Input: part model. Units: mm. Frame: model coordinates. Round coordinates to 2 decimals unless told otherwise and drop trailing zeros. Order: outer loops, then holes, each group sorted by start corner. A loop starts at its lowest first (then second) coordinate and runs counter-clockwise, first axis right, second up. Notation, with made-up numbers: (-35, 53) -> (-11, 53) arc R16 cw to (-11, 58) -> close; hole circle Ø3 at (25.5, 34). An arc over 180 degrees is marked (long way). Answer as CSV lines item,"result". Start each with the question number.
1) Section query C-C, the plane y = 15. Output: boundary loops of the cut face in (x, z).
2) Mould query, pull axis Z, two halves, no side actions, for faces 1 (the face through (-2.71, 50.7, 12.203)), 2 (the face through (10, 50.6, -3.2)). Classes: +Z half, -Z half, draft (parallel to the pull), parting line (faces both ways), or undercut.
3) Section query B-B, the plane x = 0. Output: boundary loops of the cut face in (y, z), and give its area (3 significant figures).
4) Section query A-A, the plane z = 0. Output: boundary loops of the cut face in (x, y).
5) Line query: L1, parallel to X at y = 40, z = 0; L2, parallel to Z at x = 6.5, y = 59.5. Output: solid intervals per line, ascending.
6) First-contact query: P1, Ø2, axis at x = -8, z = 3.5, coming from the +Y side; P2, Ø5, axis at x = -5.5, y = 51.5, coming from the +Z side; P3, Ø2, axis at x = -6.5, y = 54.5, coming from the +Z side (3 decimals); P4, Ø6, axis at y = 13.5, z = 0.5, coming from the +X side. Flat tips, straight axial feed; report the tip coordinate or a pass-through.
Solid Edge part; units mm, degrees
sketch "Sketch1" plane through (0, 0, 0) normal (0, 0, 1) x (1, 0, 0)
  line L0 (0, 0) -> (0, 100)
sketch "Sketch2" plane through (0, 0, 0) normal (0, -1, 0) x (1, 0, 0)
  circle A0 centre (0, 0) radius 12.5
sweep "SweptProtrusion_1" add profiles "Sketch2" path "Sketch1"
shell "Thinwall_1" thickness 2 removed faces 2 at (-8.0833, 0, 8.5833) at (-8.0833, 100, 8.5833)
sketch "Sketch3" plane through (0, 0, 0) normal (1, 0, 0) x (0, 1, 0)
  circle A0 centre (0, 0) radius 12.5
  circle A1 centre (100, 0) radius 12.5
extrude "Cutout1" cut sketch "Sketch3" along normal through all and the other way through all
properties material "Stainless steel"
Findings:
1,outline,"circle Ø25 at (0, 0); hole circle Ø21 at (0, 0)"
2,face 1,"parting line"
2,face 2,"undercut"
3,outline,"(0, -12.5) -> (100, -12.5) arc R12.5 cw to (93.22, -10.5) -> (6.78, -10.5) arc R12.5 cw to start; (0, 12.5) arc R12.5 cw to (6.78, 10.5) -> (93.22, 10.5) arc R12.5 cw to (100, 12.5) -> close"
3,area,"363 mm^2"
4,outline,"(-12.5, 12.5) -> (-10.5, 12.5) -> (-10.5, 87.5) -> (-12.5, 87.5) -> close; (10.5, 12.5) -> (12.5, 12.5) -> (12.5, 87.5) -> (10.5, 87.5) -> close"
5,L1,"x = -12.5 to -10.5, 10.5 to 12.5"
5,L2,"z = -10.68 to -8.25, 8.25 to 10.68"
6,P1,"passes through"
6,P2,"stops at z = 12.13"
6,P3,"stops at z = 11.225"
6,P4,"stops at x = 12.5"
